Verification items for the finished model (mm, model axes). A direction names the side the tool comes from. Coordinates: 2 decimals unless noted, no trailing zeros. Order: outer loops, then holes, each group sorted by start corner. A loop starts at its lowest first (then second) coordinate and runs counter-clockwise, first axis right, second up.
Q1. Cross-section at C-C, the plane z = 13.5. Record the boundary of the cut face in (x, y).
Q2. Draft check along X on faces 5 (the flat face through (-196.84, 7.61, 32.44)), 6 (the flat face through (-37, 2.5, -2)), 7 (the flat face through (-82, 0, -1)). Enter one of: pulls with the +X half, pulls with the -X half, needs draft (parallel to the pull), parting line crosses it, or undercut.
Q3. Depth check by flat-ended pin: P1, Ø3, axis at x = -3.5, y = 1.5, coming from the +Z side; P2, Ø8, axis at x = -35.5, z = -1.5, coming from the +Y side; P3, Ø12, axis at x = -192, y = 2.5, coming from the -Z side. Enter the tip coordinate at first touch or a pass-through.
Q4. Cross-section at B-B, the plane y = -3.75. Record the boundary of the cut face in (x, z), and give its area (3 significant figures).
Q5. Thickness scan on line 1 (Z direction, x = 1.5, y = 6); line 2 (Y direction, x = -9, z = -10.5); line 3 (Z direction, x = -131, y = 14.5). Record the ranges inside material, lowest first.
Q6. Cross-section at D-D, the plane y = 18. Record the boundary of the cut face in (x, z), and give its area (3 significant figures).
Q7. Cross-section at A-A, the plane x = -55.5. Record the boundary of the cut face in (y, z), and give its area (3 significant figures).
Q8. Set-up check for faces 1 (the flat face through (-24, 4.5, -3)), 2 (the flat face through (-32, 12.5, -4)), 3 (the cylindrical face through (-29.34, 1.27, -3.31)), 4 (the flat face through (-129, 8, -13.155)): record each of +Z, -Z, +X, -X, +Y, -Y from which the full face is reachable in a straight line by a thin tool's end or side.
from build123d import *

# Parameters (mm, degrees)
SKETCH_1_W          = 150
SKETCH_1_H          = 21.000000000000004
EXTRUDE_1_DEPTH     = 15
CUT_EXTRUDE_1_DEPTH = 145
SKETCH_3_R          = 5.000000000000004
CUT_EXTRUDE_2_DEPTH = 3
CUT_EXTRUDE_START   = -3
SKETCH_4_R          = 5.000000000000001
CUT_EXTRUDE_3_DEPTH = 3
SKETCH_5_R          = 2.4999999999999987
CUT_EXTRUDE_4_DEPTH = 20
SKETCH_6_R          = 5.000000000000001
CUT_EXTRUDE_5_DEPTH = 20
SKETCH_7_R          = 5.999999999999998
EXTRUDE_2_DEPTH     = 2
SKETCH_8_R          = 6.000000000000003
EXTRUDE_3_DEPTH     = 2
SKETCH_9_R          = 2.500000000000002
CUT_EXTRUDE_6_DEPTH = 20
EXTRUDE_5_DEPTH     = 15
EXTRUDE_6_DEPTH     = 5
FILLET_1_R          = 5
FILLET_2_R          = 10.5
FILLET_3_R          = 67.5
SKETCH_17_W         = 22.000000000000004
SKETCH_17_H         = 5.999999999999995
CUT_EXTRUDE_7_DEPTH = 200


with BuildPart() as part:
    # Sketch 1 → Extrude 1 (new body)
    with BuildSketch(Plane(origin=(0, 0, 0), x_dir=(1, 0, 0), z_dir=(0, 1, 0))):
        with Locations((-32.52921535893155, 2.6552587646076753)):
            Rectangle(SKETCH_1_W, SKETCH_1_H)
    extrude(amount=EXTRUDE_1_DEPTH)

    # Sketch 2 → Cut-Extrude 1 (cut)
    with BuildSketch(Plane(origin=(42.470784641068455, 0, 0), x_dir=(0, 0, -1), z_dir=(1, 0, 0))):
        Polygon((-7.844741235392326, 10.499999999999998), (13.155258764607675, 10.499999999999998), (13.155258764607675, 4.500000000000001), (-7.844741235392326, 4.5), align=None)
    extrude(amount=-CUT_EXTRUDE_1_DEPTH, mode=Mode.SUBTRACT)

    # Sketch 3 → Cut-Extrude 2 (cut)
    with BuildSketch(Plane(origin=(0, 15, 0), x_dir=(1, 0, 0), z_dir=(0, 1, 0))):
        with Locations(Location((32.47078464106845, 2.655258764607675, 0), (0, 0, 270))):
            Circle(SKETCH_3_R)
    extrude(amount=-CUT_EXTRUDE_2_DEPTH, mode=Mode.SUBTRACT)

    # Sketch 4 → Cut-Extrude 3 (cut)
    with BuildSketch(Plane(origin=(0, 0, 0), x_dir=(-1, 0, 0), z_dir=(0, -1, 0)).offset(CUT_EXTRUDE_START)):
        with Locations(Location((-32.47078464106845, 2.655258764607675, 0), (0, 0, 270))):
            Circle(SKETCH_4_R)
    extrude(amount=CUT_EXTRUDE_3_DEPTH, mode=Mode.SUBTRACT)

    # Sketch 5 → Cut-Extrude 4 (cut)
    with BuildSketch(Plane(origin=(0, 3, 0), x_dir=(-1, 0, 0), z_dir=(0, -1, 0))):
        with Locations(Location((-32.47078464106845, 2.655258764607675, 0), (0, 0, 270))):
            Circle(SKETCH_5_R)
    extrude(amount=-CUT_EXTRUDE_4_DEPTH, mode=Mode.SUBTRACT)

    # Sketch 6 → Cut-Extrude 5 (cut)
    with BuildSketch(Plane(origin=(0, 15, 0), x_dir=(1, 0, 0), z_dir=(0, 1, 0))):
        with Locations(Location((-34.295534758931545, 2.655258764607675, 0), (0, 0, 270))):
            Circle(SKETCH_6_R)
    extrude(amount=-CUT_EXTRUDE_5_DEPTH, mode=Mode.SUBTRACT)

    # Sketch 7 → Extrude 2 (add)
    with BuildSketch(Plane(origin=(0, 4.5, 1.9e-16), x_dir=(1, 0, 0), z_dir=(0, 1, 4e-17))):
        with Locations((-34.295534758931545, 2.655258764607675)):
            Circle(SKETCH_7_R)
    extrude(amount=-EXTRUDE_2_DEPTH)

    # Sketch 8 → Extrude 3 (add)
    with BuildSketch(Plane(origin=(0, 10.499999999999998, 0), x_dir=(-1, 0, 0), z_dir=(0, -1, 0))):
        with Locations((34.295534758931545, 2.655258764607675)):
            Circle(SKETCH_8_R)
    extrude(amount=-EXTRUDE_3_DEPTH)

    # Sketch 9 → Cut-Extrude 6 (cut)
    with BuildSketch(Plane(origin=(0, 12.499999999999998, 0), x_dir=(1, 0, 0), z_dir=(0, 1, 0))):
        with Locations(Location((-34.295534758931545, 2.655258764607675, 0), (0, 0, 270))):
            Circle(SKETCH_9_R)
    extrude(amount=-CUT_EXTRUDE_6_DEPTH, mode=Mode.SUBTRACT)



with BuildPart() as body_2:
    # Sketch 12 → Extrude 5 (new body)
    with BuildSketch(Plane(origin=(0, 15, 0), x_dir=(1, 0, 0), z_dir=(0, 1, 0))):
        Polygon((-107.52921535893154, -7.844741235392326), (-167.52921535893154, -7.844741235392335), (-213.49188194607015, -46.41199781658475), (-226.9904217494875, -30.32506451108624), (-175.17259027852143, 13.155258764607666), (-107.52921535893154, 13.155258764607675), align=None)
    extrude(amount=-EXTRUDE_5_DEPTH)

    # Sketch 13 → Revolve 3 (revolve)
    with BuildSketch(Plane(origin=(-148.13562673762334, 0, 124.30054975975524), x_dir=(0.6427876096865401, 0, 0.7660444431189775), z_dir=(-0.7660444431189775, 0, 0.6427876096865401))):
        with BuildLine():
            Line((-112.17628346215061, 22.5), (-112.17628346215061, -7.5))
            ThreePointArc((-112.17628346215061, -7.5), (-97.17628346215061, 7.5), (-112.17628346215061, 22.5))
        make_face()
    revolve(axis=Axis((-220.2411518477789, 22.5, 38.36853116383551), (0, -1, 0)))


with BuildPart() as part_1:
    add(part.part)

    add(body_2.part)  # Extrude 6 merges body 2
    # Sketch 14 → Extrude 6 (add)
    with BuildSketch(Plane(origin=(0, 0, -13.155258764607675), x_dir=(-1, 0, 0), z_dir=(0, 0, -1))):
        Polygon((107.52921535893154, 15), (-52.97078464106847, 14.99999999999998), (-52.97078464106847, -3.99e-14), (107.52921535893154, 0), align=None)
    extrude(amount=EXTRUDE_6_DEPTH)

    # Fillet 1
    fillet_1_edges = [part_1.edges().sort_by_distance(p)[0] for p in [
        (-107.52921535893154, 7.5, -18.155258764607673),
    ]]
    fillet(fillet_1_edges, radius=FILLET_1_R - 0.0001)  # a hair under: the kernel refuses the full size

    # Fillet 2
    fillet_2_edges = [part_1.edges().sort_by_distance(p)[0] for p in [
        (42.470784641068455, 12.75, -13.155258764607675),
    ]]
    fillet(fillet_2_edges, radius=FILLET_2_R - 0.0001)  # a hair under: the kernel refuses the full size
    fillet_2_2_edges = [part_1.edges().sort_by_distance(p)[0] for p in [
        (42.470784641068455, 2.2500000000000004, -13.155258764607675),
    ]]
    fillet(fillet_2_2_edges, radius=FILLET_2_R - 0.0001)  # a hair under: the kernel refuses the full size
    fillet_2_3_edges = [part_1.edges().sort_by_distance(p)[0] for p in [
        (42.470784641068455, 2.25, 7.844741235392326),
    ]]
    fillet(fillet_2_3_edges, radius=FILLET_2_R)
    fillet_2_4_edges = [part_1.edges().sort_by_distance(p)[0] for p in [
        (42.470784641068455, 12.75, 7.844741235392326),
    ]]
    fillet(fillet_2_4_edges, radius=FILLET_2_R)

    # Fillet 3
    fillet_3_edges = [part_1.edges().sort_by_distance(p)[0] for p in [
        (-167.52921535893154, 7.5, 7.844741235392335),
        (-175.17259027852143, 7.5, -13.155258764607666),
    ]]
    fillet(fillet_3_edges, radius=FILLET_3_R)

    # Sketch 17 → Cut-Extrude 7 (cut)
    with BuildSketch(Plane(origin=(-102.52921535893152, 0, 0), x_dir=(0, 0, -1), z_dir=(1, 0, 0))):
        with Locations((3.1552587646076753, 7.500000000000001)):
            Rectangle(SKETCH_17_W, SKETCH_17_H)
    extrude(amount=CUT_EXTRUDE_7_DEPTH, mode=Mode.SUBTRACT)


solid = part_1.part
Check values:
1. outline: (-206.94, 0) - (-170.01, 0) - (-170.01, 15) - (-206.94, 15) - close
2. face 5: pulls with the +X half
2. face 6: undercut
2. face 7: needs draft
3. P1: stops at z = 7.84
3. P2: stops at y = 15
3. P3: stops at z = -3.13
4. outline: circle Ø19.84 at (-220.24, 38.37)
4. area: 309 mm2
5. line 1: z = -18.16 to -14.16
5. line 2: y = 0 to 4.5, 10.5 to 15
5. line 3: z = -13.16 to 7.84
6. outline: circle Ø21.42 at (-220.24, 38.37)
6. area: 360 mm2
7. outline: (0, -18.16) - (15, -18.16) - (15, 7.84) - (10.5, 7.84) - (10.5, -14.16) - (4.5, -14.16) - (4.5, 7.84) - (0, 7.84) - close
7. area: 258 mm2
8. face 1: +Z, +X
8. face 2: +Y
8. face 3: -Y
8. face 4: -Z, -X, +Y, -Y
